from build123d import *

# Parameters (mm, degrees)
F0_R     = 4.9
F0_R_2   = 3.5
F1_DEPTH = 25
F0_R_3   = 7
F2_DEPTH = 3
F3_SIZE  = 2
F4_SIZE  = 1


with BuildPart() as f1:
    # F0 (on Top) → F1 (new body)
    with BuildSketch(Plane.XY):
        Circle(F0_R)
        Circle(F0_R_2, mode=Mode.SUBTRACT)
    extrude(amount=F1_DEPTH)

    # F0 (on Top) → F2 (join)
    with BuildSketch(Plane.XY):
        Circle(F0_R_3)
        Circle(F0_R, mode=Mode.SUBTRACT)
    extrude(amount=F2_DEPTH)

    # F3
    f3_edges = [f1.edges().sort_by_distance(p)[0] for p in [
        (-7, 0, 0),
    ]]
    chamfer(f3_edges, length=F3_SIZE)

    # F4
    f4_edges = [f1.edges().sort_by_distance(p)[0] for p in [
        (-3.5, 0, 25),
    ]]
    chamfer(f4_edges, length=F4_SIZE)


solid = f1.part
Geometry check sheet. Reference: the model listing, model coordinates, mm. Round coordinates to 2 decimals unless told otherwise and drop trailing zeros. Loops run counter-clockwise (first coordinate to the right, second up) from the corner with the lowest first, then second, coordinate; pieces in that order, holes last.
Item 1: Cross-section at C-C on z = 15.75. Record the boundary of the cut face in (x, y).
Item 2: Gauge pin test, flat ends, axial feed: pin 1 (8 mm diameter, centred on x = 4.5, z = 20.5, fed in from -Y); pin 2 (2 mm diameter, centred on x = -3.5, y = 4.5, fed in from -Z); pin 3 (1.5 mm diameter, centred on x = 5, y = 4, fed in from -Z); pin 4 (5 mm diameter, centred on y = 3, z = 13, fed in from -X). Record the tip position at first contact, or that the pin passes through.
Item 3: Thickness scan on line 1 (Y direction, x = 0, z = 7.5); line 2 (Y direction, x = 2.75, z = 14.75); line 3 (X direction, y = -2.5, z = 17). Record the ranges inside material, lowest first.
Item 4: Cross-section at A-A on y = 0. Record the boundary of the cut face in (x, z).
Item 5: Mould release check, pull along Y, two halves, no side actions. Record for faces 1 (the cylindrical face through (3.233, -1.341, 11.832)), 2 (the flat face through (2.2, -3.3, 0)), 3 (the cylindrical face through (6.466, -2.681, 2.493)): pulls with the +Y half, pulls with the -Y half, needs draft (parallel to the pull), parting line crosses it, or undercut.
Answer sheet:
1. outline: circle Ø9.8 at (0, 0); hole circle Ø7 at (0, 0)
2. pin 1: stops at y = -4.87
2. pin 2: stops at z = 0
2. pin 3: stops at z = 0.65
2. pin 4: stops at x = -4.87
3. line 1: y = -4.9 to -3.5, 3.5 to 4.9
3. line 2: y = -4.06 to -2.17, 2.17 to 4.06
3. line 3: x = -4.21 to -2.45, 2.45 to 4.21
4. outline: (-7, 2) - (-5, 0) - (-3.5, 0) - (-3.5, 24) - (-4.5, 25) - (-4.9, 25) - (-4.9, 3) - (-7, 3) - close; (3.5, 0) - (5, 0) - (7, 2) - (7, 3) - (4.9, 3) - (4.9, 25) - (4.5, 25) - (3.5, 24) - close
5. face 1: undercut
5. face 2: needs draft
5. face 3: parting line crosses it
